```python
from build123d import *

# Parameters (mm, degrees)
SKETCH1_R           = 1.25
BOSS_EXTRUDE1_DEPTH = 4
SKETCH2_R           = 2.5
BOSS_EXTRUDE2_DEPTH = 2
SKETCH3_R           = 1.25
SKETCH3_R_2         = 1
BOSS_EXTRUDE3_DEPTH = 5
FILLET1_R           = 1


with BuildPart() as part:
    # Sketch1 → Boss-Extrude1 (new body)
    with BuildSketch(Plane(origin=(0, 0, 0), x_dir=(1, 0, 0), z_dir=(0, 1, 0))):
        Circle(SKETCH1_R)
    extrude(amount=BOSS_EXTRUDE1_DEPTH)

    # Sketch2 → Boss-Extrude2 (add)
    with BuildSketch(Plane(origin=(0, 4, 0), x_dir=(1, 0, 0), z_dir=(0, 1, 0))):
        Circle(SKETCH2_R)
    extrude(amount=BOSS_EXTRUDE2_DEPTH)

    # Sketch3 → Boss-Extrude3 (add)
    with BuildSketch(Plane(origin=(0, 6, 0), x_dir=(1, 0, 0), z_dir=(0, 1, 0))):
        Circle(SKETCH3_R)
        Circle(SKETCH3_R_2, mode=Mode.SUBTRACT)
    extrude(amount=BOSS_EXTRUDE3_DEPTH)

    # Fillet1
    fillet1_edges = [part.edges().sort_by_distance(p)[0] for p in [
        (-1.25, 0, 0),
    ]]
    fillet(fillet1_edges, radius=FILLET1_R)


solid = part.part
```
Geometry: final body of the model. Coordinates: model frame, mm. A direction names the side the tool comes from. Coordinates: 2 decimals unless noted, no trailing zeros. Write each loop counter-clockwise with the first axis right and the second up, starting at its lowest first coordinate (ties: lowest second). Pieces come first, ordered by that corner, then holes. Notation, with made-up numbers: M -5,4 L 45,4 A8 ccw 45,11 Z; hole C 53,-27 d11. An arc over 180 degrees is marked long. Use CSV: the item, a comma, the result in double quotes. Start each with the question number.
1. Cut plane C-C on z = 2.15. Return the cut outline in (x, y).
2. Ray query, probe 1 along Z at (x, y) = (0, 7.2); probe 2 along Y at (x, z) = (-2.05, -0.1). Return the intervals inside material, ascending.
3. First-contact query: P1, Ø2, axis at x = -1.5, z = -0.5, coming from the +Y side; P2, Ø3, axis at y = 9, z = 1, coming from the +X side. Flat tips, straight axial feed; report the tip coordinate or a pass-through.
4. Mould query, pull axis X, two halves, no side actions, for faces 1 (the face through (-1, 4, 1)), 2 (the face through (-0.27, 8.46, 1.22)), 3 (the face through (0, 8, 1)), 4 (the face through (0, 6, 0)). Classes: pulls with the +X half, pulls with the -X half, needs draft (parallel to the pull), parting line crosses it, or undercut.
5. Cut plane A-A on y = 8.75. Return the cut outline in (x, z).
6. Reachability of faces 5 (the face through (-1, 6, 1)), 6 (the face through (-0.54, 4.99, 2.44)), 7 (the face through (-0.27, 2.48, 1.22)) from +Z, -Z, +X, -X, +Y, -Y: full face, straight path, thin tool, end or side. Return the list, or none.
7. Cut plane B-B on y = 5.5. Return the cut outline in (x, z).
8. Cut plane D-D on x = 1.45. Return the cut outline in (y, z).
Entries:
1,outline,"M -1.28,4 L 1.28,4 L 1.28,6 L -1.28,6 Z"
2,probe 1,"-1.25 to -1, 1 to 1.25"
2,probe 2,"4 to 6"
3,P1,"y = 11"
3,P2,"x = 1.25"
4,face 1,"needs draft"
4,face 2,"parting line crosses it"
4,face 3,"undercut"
4,face 4,"undercut"
5,outline,"C 0,0 d2.5; hole C 0,0 d2"
6,face 5,"+Y"
6,face 6,"+Y, -Y"
6,face 7,"-Y"
7,outline,"C 0,0 d5"
8,outline,"M 4,-2.04 L 6,-2.04 L 6,2.04 L 4,2.04 Z"
